Could you check a few things on this model? Use its own coordinates, in mm. A direction names the side the tool comes from. Coordinates: 2 decimals unless noted, no trailing zeros. Order: outer loops, then holes, each group sorted by start corner. A loop starts at its lowest first (then second) coordinate and runs counter-clockwise, first axis right, second up. Notation, with made-up numbers: (-38.5, 31) -> (-9.5, 31) arc R32 ccw to (-9.5, 65) -> close; hole circle Ø5 at (7.25, -19.5). An arc over 180 degrees is marked (long way). Put each result on its own line as item: value. Start each with the question number.
Q1. We'd pull the mould along Y, two halves only. Please class faces 1 (the face through (145.25, 53.78, 13.38)), 2 (the face through (147, 62, 15.78)), 3 (the face through (146.73, 55.78, 13.33)), 4 (the face through (147, 62, 9.78)): +Y half, -Y half, draft (parallel to the pull), parting line (faces both ways), or undercut.
Q2. If we section it at B-B (y = 64): Please give me the cut outline in (x, z).
Q3. If we section it at C-C (z = 13.28): Please give me the cut outline in (x, y).
Q4. If we section it at A-A (x = 146.6): Please give me the cut outline in (y, z), and give its area (3 significant figures).
Q5. Will these pins go through, and if not, where does the flat tip stop? pin 1 (2.5 mm diameter, centred on y = 63, z = 15, fed in from +X); pin 2 (0.8 mm diameter, centred on x = 146.5, y = 63.5, fed in from -Z).
Q6. For faces 5 (the face through (146.73, 69.78, 13.2)), 6 (the face through (146.73, 54.78, 13.36)), 7 (the face through (147, 62, 10.78)), 8 (the face through (147, 62, 16.78)), 9 (the face through (145, 62, 13)), which set-ups out of +Z, -Z, +X, -X, +Y, -Y let a thin tool reach every point of the face, with its end or its side?
Q7. Please list where these lines run through material, in increasing order: line 1 along Z through (x, y) = (146.5, 61.25); line 2 along X through (y, z) = (66, 13); line 3 along Y through (x, z) = (147.8, 12.5).
Q8. If we section it at D-D (y = 69.5): Please give me the cut outline in (x, z).
from build123d import *

# Parameters (mm, degrees)
EXTRUDE002_DEPTH = 0.5
EXTRUDE001_DEPTH = 3


with BuildPart() as extrude002:
    # Sketch002 → Extrude002 (new body)
    with BuildSketch(Plane.YZ):
        with BuildLine():
            Line((58.28, 3.78), (66.28, 3.78))
            ThreePointArc((66.28, 3.78), (70.780004, 8.28), (66.28, 12.78))
            Line((58.28, 12.78), (66.28, 12.78))
            ThreePointArc((58.28, 12.78), (53.779996, 8.28), (58.28, 3.78))
        make_face()
    extrude(amount=EXTRUDE002_DEPTH)


with BuildPart() as extrude002_1:
    # Extrude002 placement: moved
    add(extrude002.part.moved(Location((145, 0, 5))))


with BuildPart() as usb_tap:
    # Sketch001 → Extrude001 (new body)
    with BuildSketch(Plane.YZ):
        with BuildLine():
            Line((58.28, 4.78), (66.28, 4.78))
            ThreePointArc((66.28, 4.78), (69.779995, 8.28), (66.28, 11.78))
            Line((58.28, 11.78), (66.28, 11.78))
            ThreePointArc((58.28, 11.78), (54.779995, 8.28), (58.28, 4.78))
        make_face()
        with BuildLine():
            ThreePointArc((58.279995, 10.78), (55.779995, 8.28), (58.279995, 5.78))
            Line((58.279995, 5.78), (66.279995, 5.78))
            ThreePointArc((66.279995, 5.78), (68.779995, 8.28), (66.279995, 10.78))
            Line((58.279995, 10.78), (66.279995, 10.78))
        make_face(mode=Mode.SUBTRACT)
    extrude(amount=EXTRUDE001_DEPTH)


with BuildPart() as usb_tap_1:
    # Extrude001 placement: moved
    add(usb_tap.part.moved(Location((145, 0, 5))))

    # Fusion062: union Extrude002
    add(extrude002_1.part)


solid = usb_tap_1.part
The answers:
1. face 1: -Y half
1. face 2: undercut
1. face 3: undercut
1. face 4: draft
2. outline: (145, 8.78) -> (145.5, 8.78) -> (145.5, 9.78) -> (148, 9.78) -> (148, 10.78) -> (145.5, 10.78) -> (145.5, 15.78) -> (148, 15.78) -> (148, 16.78) -> (145.5, 16.78) -> (145.5, 17.78) -> (145, 17.78) -> close
3. outline: (145, 53.78) -> (145.5, 53.78) -> (145.5, 54.78) -> (148, 54.78) -> (148, 55.78) -> (145.5, 55.78) -> (145.5, 68.78) -> (148, 68.78) -> (148, 69.78) -> (145.5, 69.78) -> (145.5, 70.78) -> (145, 70.78) -> close
4. outline: (58.28, 9.78) -> (66.28, 9.78) arc R3.5 ccw to (66.28, 16.78) -> (58.28, 16.78) arc R3.5 ccw to start; hole (58.28, 10.78) -> (66.28, 10.78) arc R2.5 ccw to (66.28, 15.78) -> (58.28, 15.78) arc R2.5 ccw to start
4. area: 34.8 mm^2
5. pin 1: x = 148
5. pin 2: z = 9.78
6. face 5: +X, +Y
6. face 6: +X, -Y
6. face 7: +X
6. face 8: +Z, +X, +Y, -Y
6. face 9: +Z, -Z, -X, +Y, -Y
7. line 1: 9.78 to 10.78, 15.78 to 16.78
7. line 2: 145 to 145.5
7. line 3: 54.87 to 55.9, 68.66 to 69.69
8. outline: (145, 10.14) -> (145.5, 10.14) -> (145.5, 11.91) -> (148, 11.91) -> (148, 14.65) -> (145.5, 14.65) -> (145.5, 16.42) -> (145, 16.42) -> close
